The listing builds one solid part. Answer for the finished solid, in the listing's coordinates (mm). A direction names the side the tool comes from. Round coordinates to 2 decimals unless told otherwise and drop trailing zeros. Loops run counter-clockwise (first coordinate to the right, second up) from the corner with the lowest first, then second, coordinate; pieces in that order, holes last. Notation, with made-up numbers: (83.5, 21.25) -> (134.5, 21.25) arc R34 ccw to (134.5, 59.25) -> close; hole circle Ø7 at (89.5, 12). An arc over 180 degrees is marked (long way). Write each question's results on one line, items separated by ' | '. Start each with the question number.
(1) Straight lines are drawn through the part: probe 1 along Z at (x, y) = (22.5, 11.5); probe 2 along Z at (x, y) = (23, 24.5); probe 3 along Y at (x, z) = (20.5, 17.5). For each, find the intervals that lie inside material, in ascending order.
(2) The part is cut by section D-D (y = -40). Determine the outline of the cut face in (x, z).
(3) The part is cut by section A-A (y = 21.5). Determine the outline of the cut face in (x, z), plus the area to 4 significant figures.
(4) For faces 1 (the face through (19, 25, 0)), 2 (the face through (15, -40, 32)), 3 (the face through (24, -20, 0)), determine the directions among +Z, -Z, +X, -X, +Y, -Y from which every point of the face is accessible in a straight line to the end or side of a thin tool.
(5) The part is cut by section C-C (x = 8). Determine the outline of the cut face in (y, z).
(6) Determine the mould class of faces 4 (the face through (19, -25, -5)), 5 (the face through (20, 25, 25)), 6 (the face through (21, 38, 36)) for opening direction X: released by +X, released by -X, zero draft, split by the parting line, or undercut.
(7) The part is cut by section B-B (z = -0.5). Determine the outline of the cut face in (x, y), plus the area to 3 significant figures.
(8) Flat-ended cylindrical pins translate along their axes: pin 1 (2 mm diameter, centred on y = -24.5, z = -4, fed in from +X); pin 2 (6 mm diameter, centred on x = 33.5, z = 4.5, fed in from -Y); pin 3 (16 mm diameter, centred on y = -5.5, z = -1.5, fed in from +X). Find the tip coordinate at first contact, or state that the pin passes through.
```python
from build123d import *

# Parameters (mm, degrees)
SKETCH1_W           = 30
SKETCH1_H           = 60
BOSS_EXTRUDE1_DEPTH = 39
SKETCH2_W           = 20
SKETCH2_H           = 40
CUT_EXTRUDE1_DEPTH  = 30
SKETCH3_R           = 2
CUT_EXTRUDE2_DEPTH  = 20
SKETCH4_W           = 10
SKETCH4_H           = 20
CUT_EXTRUDE3_DEPTH  = 10
SKETCH5_W           = 39
SKETCH5_H           = 60
BOSS_EXTRUDE2_DEPTH = 25
SKETCH6_W           = 20
SKETCH6_H           = 50
CUT_EXTRUDE4_DEPTH  = 39
SKETCH7_W           = 39
SKETCH7_H           = 8
BOSS_EXTRUDE3_DEPTH = 20
SKETCH8_W           = 39
SKETCH8_H           = 8
BOSS_EXTRUDE4_DEPTH = 20
SKETCH9_R           = 2.5
CUT_EXTRUDE5_DEPTH  = 8


with BuildPart() as part:
    # Sketch1 → Boss-Extrude1 (new body)
    with BuildSketch(Plane(origin=(0, 0, 0), x_dir=(0, 0, -1), z_dir=(1, 0, 0))):
        Rectangle(SKETCH1_W, SKETCH1_H)
    extrude(amount=BOSS_EXTRUDE1_DEPTH)

    # Sketch2 → Cut-Extrude1 (cut)
    with BuildSketch(Plane(origin=(39, 0, 0), x_dir=(0, 0, -1), z_dir=(1, 0, 0))):
        Rectangle(SKETCH2_W, SKETCH2_H)
    extrude(amount=-CUT_EXTRUDE1_DEPTH, mode=Mode.SUBTRACT)

    # Sketch3 → Cut-Extrude2 (cut)
    with BuildSketch(Plane(origin=(39, 0, 0), x_dir=(0, 0, -1), z_dir=(1, 0, 0))):
        with Locations((-4.925, 24.71)):
            Circle(SKETCH3_R)
        with Locations((4.925, 24.71)):
            Circle(SKETCH3_R)
        with Locations(Location((4.925, -24.71, 0), (0, 0, 180))):
            Circle(SKETCH3_R)
        with Locations(Location((-4.925, -24.71, 0), (0, 0, 180))):
            Circle(SKETCH3_R)
    extrude(amount=-CUT_EXTRUDE2_DEPTH, mode=Mode.SUBTRACT)

    # Sketch4 → Cut-Extrude3 (cut)
    with BuildSketch(Plane.XZ.offset(-20)):
        with Locations((14, 0)):
            Rectangle(SKETCH4_W, SKETCH4_H)
    extrude(amount=-CUT_EXTRUDE3_DEPTH, mode=Mode.SUBTRACT)

    # Sketch5 → Boss-Extrude2 (add)
    with BuildSketch(Plane.XY.offset(15)):
        with Locations((19.5, 0)):
            Rectangle(SKETCH5_W, SKETCH5_H)
    extrude(amount=BOSS_EXTRUDE2_DEPTH)

    # Sketch6 → Cut-Extrude4 (cut)
    with BuildSketch(Plane(origin=(39, 0, 0), x_dir=(0, 0, -1), z_dir=(1, 0, 0))):
        with Locations((-25, 0)):
            Rectangle(SKETCH6_W, SKETCH6_H)
    extrude(amount=-CUT_EXTRUDE4_DEPTH, mode=Mode.SUBTRACT)

    # Sketch7 → Boss-Extrude3 (add)
    with BuildSketch(Plane(origin=(0, -30, 0), x_dir=(-1, 0, 0), z_dir=(0, -1, 0))):
        with Locations((-19.5, -36)):
            Rectangle(SKETCH7_W, SKETCH7_H)
    extrude(amount=BOSS_EXTRUDE3_DEPTH)

    # Sketch8 → Boss-Extrude4 (add)
    with BuildSketch(Plane(origin=(0, 30, 0), x_dir=(1, 0, 0), z_dir=(0, 1, 0))):
        with Locations((19.5, -36)):
            Rectangle(SKETCH8_W, SKETCH8_H)
    extrude(amount=BOSS_EXTRUDE4_DEPTH)

    # Sketch9 → Cut-Extrude5 (cut)
    with BuildSketch(Plane(origin=(0, 0, 32), x_dir=(-1, 0, 0), z_dir=(0, 0, -1))):
        with Locations((-19.5, -40)):
            Circle(SKETCH9_R)
        with Locations((-19.5, 40)):
            Circle(SKETCH9_R)
    extrude(amount=-CUT_EXTRUDE5_DEPTH, mode=Mode.SUBTRACT)


solid = part.part
```
Checked values:
1) probe 1: z = -15 to -10, 10 to 15, 35 to 40 | probe 2: z = -15 to -6.91, -2.94 to 2.94, 6.91 to 15, 35 to 40 | probe 3: y = -30 to -25, 25 to 30
2) outline: (0, 32) -> (17, 32) -> (17, 40) -> (0, 40) -> close; (22, 32) -> (39, 32) -> (39, 40) -> (22, 40) -> close
3) outline: (0, -15) -> (39, -15) -> (39, 15) -> (0, 15) -> close; (0, 35) -> (39, 35) -> (39, 40) -> (0, 40) -> close; hole (9, -10) -> (19, -10) -> (19, 10) -> (9, 10) -> close | area: 1,165 mm2
4) face 1: +Y | face 2: -Z, +X, -X, -Y | face 3: +X
5) outline: (-50, 32) -> (-30, 32) -> (-30, -15) -> (30, -15) -> (30, 32) -> (50, 32) -> (50, 40) -> (-50, 40) -> close; hole (-25, 15) -> (25, 15) -> (25, 35) -> (-25, 35) -> close
6) face 4: released by +X | face 5: zero draft | face 6: undercut
7) outline: (0, -30) -> (39, -30) -> (39, -20) -> (9, -20) -> (9, 30) -> (0, 30) -> close; (19, 20) -> (39, 20) -> (39, 30) -> (19, 30) -> close | area: 1,040 mm2
8) pin 1: stops at x = 19 | pin 2: stops at y = -30 | pin 3: stops at x = 9
